Here's how the part is built. I have some questions about the finished solid (model axes, mm). Round coordinates to 2 decimals unless told otherwise and drop trailing zeros. Order: outer loops, then holes, each group sorted by start corner. A loop starts at its lowest first (then second) coordinate and runs counter-clockwise, first axis right, second up. Notation, with made-up numbers: (-15, 73.25) -> (-2, 73.25) arc R21 ccw to (-2, 101.25) -> close; hole circle Ø10 at (59, 20.25). An arc over 180 degrees is marked (long way). Use a Markdown table: item, result. Add a question column.
from build123d import *

# Parameters (mm, degrees)
F1_DEPTH = 150
F3_D     = 4.4
F3_DEPTH = 14.1
F3_TIP   = 1.3218933619


with BuildPart() as f1:
    # F0 (on Front) → F1 (new body)
    with BuildSketch(Plane.XZ):
        Polygon((10, 39.4974746831), (0, 49.4974746831), (0, 0), (10, 0), align=None)
    extrude(amount=F1_DEPTH)

    # F3
    with Locations(Plane(origin=(24.7487373415, 0, 24.7487373415), x_dir=(0.7071067812, 0, -0.7071067812), z_dir=(0.7071067812, 0, 0.7071067812))):
        with Locations((-30, -130), (-30, -20)):
            Hole(F3_D / 2, depth=F3_DEPTH)
            with Locations((0, 0, -(F3_DEPTH + F3_TIP / 2))):  # 118° drill point
                Cone(0, F3_D / 2, F3_TIP, mode=Mode.SUBTRACT)


solid = f1.part
(1) If we mould it in two halves opening along Y, with no side actions, what happens to faces 1 (the flat face through (5, -150, 25)), 2 (the flat face through (5.1, -74, 44.4)), 3 (the cylindrical face through (3.05, -19.9, 42.37))? For each: pulls with the +Y half, pulls with the -Y half, needs draft (parallel to the pull), parting line crosses it, or undercut.
(2) I want a section at A-A on y = -93.5. List the corners of the cut face in (x, z) for me.
(3) I'm going to push a flat-ended pin straight in: P1, Ø1, axis at x = 1, y = -87, coming from the +Z side. Where does the tip first touch, or does it pass through?
(4) Please list where these lines run through material, in increasing order: probe 1 along Y at (x, z) = (2, 47); probe 2 along Z at (x, y) = (2, -38.5); probe 3 along Z at (x, y) = (1.5, -80). Write a range as from..to.
Output:
| question | item | result |
|---|---|---|
| 1 | face 1 | pulls with the -Y half |
| 1 | face 2 | needs draft |
| 1 | face 3 | undercut |
| 2 | outline | (0, 0) -> (10, 0) -> (10, 39.5) -> (0, 49.5) -> close |
| 3 | P1 | z = 49 |
| 4 | probe 1 | -150..-131.24, -128.76..-21.24, -18.76..0 |
| 4 | probe 2 | 0..47.5 |
| 4 | probe 3 | 0..48 |
